from build123d import *

# Parameters (mm, degrees)
SKETCH3_R               = 8
BOSS_EXTRUDE1_DEPTH     = 21.052631579
CUT_EXTRUDE1_DEPTH      = 11.160006171
CUT_EXTRUDE1_DEPTH_BACK = 11.160006171
CUT_EXTRUDE2_DEPTH      = 11.146902499
CUT_EXTRUDE2_DEPTH_BACK = 11.1469025
BOSS_EXTRUDE3_DEPTH     = 1.2
SKETCH8_R               = 1.6
SKETCH8_R_2             = 1.4
CUT_EXTRUDE3_DEPTH      = 25.395624714
CUT_EXTRUDE3_DEPTH_BACK = 2.513887999
CUT_EXTRUDE4_DEPTH      = 23.566519578


with BuildPart() as part:
    # Sketch3 → Boss-Extrude1 (new body)
    with BuildSketch(Plane(origin=(-12.082314344, 217.636022384, 0), x_dir=(-0.994665758, -0.103150523, 0), z_dir=(0.103150523, -0.994665758, 0))):
        Circle(SKETCH3_R)
    extrude(amount=BOSS_EXTRUDE1_DEPTH)

    # Sketch4 → Cut-Extrude1 (cut, two sides)
    with BuildSketch(Plane(origin=(10.375761543, 1.076004901, 0), x_dir=(0.103150523, -0.994665758, 0), z_dir=(-0.994665758, -0.103150523, 0))) as cut_extrude1_sk:
        with BuildLine():
            Line((-217.721396158, 8), (-213.721396158, 8))
            ThreePointArc((-213.721396158, 8), (-217.59367935, 0), (-213.721396158, -8))
            Line((-213.721396158, -8), (-217.721396158, -8))
            Line((-217.721396158, -8), (-217.721396158, 8))
        make_face()
    extrude(amount=CUT_EXTRUDE1_DEPTH, mode=Mode.SUBTRACT)
    extrude(cut_extrude1_sk.sketch, amount=-CUT_EXTRUDE1_DEPTH_BACK, mode=Mode.SUBTRACT)

    # Sketch5 → Cut-Extrude2 (cut, two sides)
    with BuildSketch(Plane(origin=(10.375761543, 1.076004901, 0), x_dir=(0.103150523, -0.994665758, 0), z_dir=(-0.994665758, -0.103150523, 0))) as cut_extrude2_sk:
        Polygon((-196.668764579, 0), (-204.668764579, 8), (-196.668764579, 8), align=None)
    extrude(amount=CUT_EXTRUDE2_DEPTH, mode=Mode.SUBTRACT)
    extrude(cut_extrude2_sk.sketch, amount=-CUT_EXTRUDE2_DEPTH_BACK, mode=Mode.SUBTRACT)

    # Sketch7 → Boss-Extrude3 (add, symmetric)
    with BuildSketch(Plane(origin=(10.375761543, 1.076004901, 0), x_dir=(0.103150523, -0.994665758, 0), z_dir=(-0.994665758, -0.103150523, 0))):
        with BuildLine():
            Line((-198.648663566, 1.979898987), (-196.668764579, 0))
            Line((-196.668764579, 0), (-196.668764579, -2.8))
            Line((-196.668764579, -2.8), (-194.243893448, 1.4))
            ThreePointArc((-194.243893448, 1.4), (-196.303291241, 2.776045612), (-198.648663566, 1.979898987))
        make_face()
    extrude(amount=BOSS_EXTRUDE3_DEPTH, both=True)

    # Sketch8 → Cut-Extrude3 (cut, two sides)
    with BuildSketch(Plane(origin=(-12.082314344, 217.636022384, 0), x_dir=(-0.994665758, -0.103150523, 0), z_dir=(0.103150523, -0.994665758, 0))) as cut_extrude3_sk:
        with Locations((-3.6, 3)):
            Circle(SKETCH8_R)
        with Locations((3.6, 3)):
            Circle(SKETCH8_R)
        with Locations((0, -5.5)):
            Circle(SKETCH8_R_2)
    extrude(amount=CUT_EXTRUDE3_DEPTH, mode=Mode.SUBTRACT)
    extrude(cut_extrude3_sk.sketch, amount=-CUT_EXTRUDE3_DEPTH_BACK, mode=Mode.SUBTRACT)

    # Sketch9 → Cut-Extrude4 (cut, through all)
    with BuildSketch(Plane(origin=(-20.286485929, 195.619685742, 0), x_dir=(0.994665758, 0.103150523, 0), z_dir=(0.103150523, -0.994665758, 0))):
        with BuildLine():
            Line((7.933405986, -7.6), (12.929404385, -7.6))
            ThreePointArc((12.929404385, -7.6), (10.431405186, -8), (7.933405986, -7.6))
        make_face()
        with BuildLine():
            Line((7.933405986, 7.6), (12.929404385, 7.6))
            ThreePointArc((12.929404385, 7.6), (10.431405186, 8), (7.933405986, 7.6))
        make_face()
    extrude(amount=-CUT_EXTRUDE4_DEPTH, mode=Mode.SUBTRACT)


solid = part.part
CAD build for the part. Positions are in the model's coordinates, mm. A direction names the side the tool comes from. Give positions to 0.01 mm unless a question says otherwise; leave off trailing zeros. Order: outer loops, then holes, each group sorted by start corner. A loop starts at its lowest first (then second) coordinate and runs counter-clockwise, first axis right, second up. Notation, with made-up numbers: (65, 77) - (88, 77) arc R18 ccw to (88, 112) - close; hole circle Ø1 at (45.5, 82). An arc over 180 degrees is marked (long way). Write each question's results on one line, items separated by ' | '.
1. Pin check, flat tips, straight feed: pin 1 (5 mm diameter, centred on x = -5, z = -4, fed in from -Y); pin 2 (3 mm diameter, centred on y = 208.5, z = 1.5, fed in from -X); pin 3 (1.5 mm diameter, centred on x = -11, z = -1.5, fed in from -Y). Stop position of each tip, or through.
Calculated:
pin 1: stops at y = 196.95 | pin 2: stops at x = -19.28 | pin 3: stops at y = 195.39
2. 3-axis set-ups, long thin cutter, end or side, ignore diameter. For faces 4 (the face through (-11, 209, 7.6)), 5 (the face through (-11.085, 196.381, 0.661)), 6 (the face through (-8.697, 196.629, 0.661)): which of +Z, -Z, +X, -X, +Y, -Y reach the whole face in a straight line?
Calculated:
face 4: +Z, +X, -X, +Y, -Y | face 5: +Z, -Y | face 6: +Z, +X
3. Pull direction Z, two halves, no side cores. Call faces 1 (the face through (-3.05, 208.07, -0.14)), 2 (the face through (-10.99, 208.83, 4.11)), 3 (the face through (-9.89, 196.3, 2.77)): released by +Z, released by -Z, zero draft, split by the parting line, or undercut.
Calculated:
face 1: split by the parting line | face 2: undercut | face 3: released by +Z
4. Saw through at C-C on y = 215.25. Count the separate pieces of the cut face and the enclosed holes in it, and give its area (3 significant figures).
Calculated:
separate pieces: 1 | enclosed holes: 2 | area: 158 mm2
5. Probe L1, parallel to X at y = 200.75, z = -3; L2, parallel to X at y = 203.5, z = -2.75; L3, parallel to Z at x = -11.25, y = 204.25. List the from-to ranges inside material, lowest first. Write a range as from..to.
Calculated:
L1: x = -17.79..-15.56, -12.34..-8.32, -5.1..-2.88 | L2: x = -18.17..-15.82, -12.65..-8.59, -5.41..-3.06 | L3: z = -7.6..4.21, 6.79..7.6
6. Saw through at A-A on z = 6.5. List the corners of the cut face in (x, y), and give its area (3 significant figures).
Calculated:
outline: (-16.47, 214.7) - (-15.22, 202.68) - (-11.56, 203.06) - (-12.8, 215.08) - close; (-10.85, 215.28) - (-9.61, 203.26) - (-5.94, 203.64) - (-7.19, 215.66) - close | area: 89.0 mm2
7. Saw through at B-B on z = -0.75. List the corners of the cut face in (x, y), and give its area (3 significant figures).
Calculated:
outline: (-19.99, 216.66) - (-17.83, 195.87) - (-11.1, 196.57) - (-10.98, 195.39) - (-8.6, 195.64) - (-8.72, 196.82) - (-1.99, 197.52) - (-4.14, 218.3) - close | area: 336 mm2
